For this review, take the finished solid that the model builds, in its own axes (mm). A direction names the side the tool comes from. Coordinates: 2 decimals unless noted, no trailing zeros. Loops run counter-clockwise (first coordinate to the right, second up) from the corner with the lowest first, then second, coordinate; pieces in that order, holes last.
```python
from build123d import *

# Parameters (mm, degrees)
EXTRUDE_1_DEPTH          = 2
SKETCH_2_R               = 1.5
CUT_EXTRUDE_1_DEPTH      = 56.208694967
MIRROR_2_COPY_1_SKETCH_R = 1.5
MIRROR_2_COPY_1_DEPTH    = 56.208694967
CUT_EXTRUDE_2_DEPTH      = 56.208694967
PATTERN_LINEAR_1_COUNT   = 6
PATTERN_LINEAR_1_PITCH   = 12
SKETCH_4_W               = 60
SKETCH_4_H               = 2
EXTRUDE_2_DEPTH          = 8
CUT_EXTRUDE_3_DEPTH      = 56.208694967
FILLET_1_R               = 3


with BuildPart() as part:
    # 草图1 → 凸台-拉伸1 (new body)
    with BuildSketch(Plane(origin=(0, 0, 0), x_dir=(1, 0, 0), z_dir=(0, 1, 0))):
        Polygon((-38, -30), (-38, -40), (38, -40), (38, -30), (30, -30), (30, 30), (38, 30), (38, 40), (-38, 40), (-38, 30), (-30, 30), (-30, -30), align=None)
    extrude(amount=EXTRUDE_1_DEPTH)

    # 草图2 → 切除-拉伸1 (cut, through all)
    with BuildSketch(Plane(origin=(0, 2, 0), x_dir=(1, 0, 0), z_dir=(0, 1, 0))):
        with Locations(Location((-34, 35, 0), (0, 0, 270))):
            Circle(SKETCH_2_R)
    cut_extrude_1 = extrude(amount=-CUT_EXTRUDE_1_DEPTH, mode=Mode.SUBTRACT)

    # 镜向1: 切除-拉伸1 across plane
    add(cut_extrude_1.mirror(Plane(origin=(0, 0, 0), x_dir=(0, 0, 1), z_dir=(1, 0, 0))), mode=Mode.SUBTRACT)

    # 镜向2: 切除-拉伸1 across plane
    add(cut_extrude_1.mirror(Plane.XY), mode=Mode.SUBTRACT)

    # 镜向2 copy 1 sketch → 镜向2 copy 1 (cut, through all)
    with BuildSketch(Plane(origin=(0, 2, 0), x_dir=(-1, 0, 0), z_dir=(0, 1, 0))):
        with Locations(Location((-34, 35, 0), (0, 0, 270))):
            Circle(MIRROR_2_COPY_1_SKETCH_R)
    extrude(amount=-MIRROR_2_COPY_1_DEPTH, mode=Mode.SUBTRACT)

    # 草图3 → 切除-拉伸2 (cut, through all)
    with BuildSketch(Plane(origin=(0, 2, 0), x_dir=(1, 0, 0), z_dir=(0, 1, 0))):
        with BuildLine():
            Line((-24, 34), (24, 34))
            ThreePointArc((24, 34), (28.5, 29.5), (24, 25))
            Line((24, 25), (-24, 25))
            ThreePointArc((-24, 25), (-28.5, 29.5), (-24, 34))
        make_face()
    cut_extrude_2 = extrude(amount=-CUT_EXTRUDE_2_DEPTH, mode=Mode.SUBTRACT)

    # 阵列(线性)1: 切除-拉伸2 ×6
    with Locations(*[(0, 0, i * PATTERN_LINEAR_1_PITCH) for i in range(1, PATTERN_LINEAR_1_COUNT)]):
        add(cut_extrude_2, mode=Mode.SUBTRACT)

    # 草图4 → 凸台-拉伸2 (add)
    with BuildSketch(Plane(origin=(30, 0, 0), x_dir=(0, 0, -1), z_dir=(1, 0, 0))):
        with Locations((0, 1)):
            Rectangle(SKETCH_4_W, SKETCH_4_H)
    extrude_2 = extrude(amount=EXTRUDE_2_DEPTH)

    # 镜向3: 凸台-拉伸2 across plane
    add(extrude_2.mirror(Plane(origin=(0, 0, 0), x_dir=(0, 0, 1), z_dir=(1, 0, 0))))

    # 草图6 → 切除-拉伸3 (cut, through all)
    with BuildSketch(Plane(origin=(0, 2, 0), x_dir=(1, 0, 0), z_dir=(0, 1, 0))):
        with BuildLine():
            Line((-38, 4), (-34, 4))
            ThreePointArc((-34, 4), (-30, 0), (-34, -4))
            Line((-34, -4), (-38, -4))
            Line((-38, -4), (-38, 4))
        make_face()
        with BuildLine():
            Line((38, -4), (38, 4))
            Line((38, 4), (34, 4))
            ThreePointArc((34, 4), (30, 0), (34, -4))
            Line((34, -4), (38, -4))
        make_face()
    extrude(amount=-CUT_EXTRUDE_3_DEPTH, mode=Mode.SUBTRACT)

    # 圆角1
    fillet_1_edges = [part.edges().sort_by_distance(p)[0] for p in [
        (-38, 1, 4),
        (-38, 1, -4),
        (38, 1, -4),
        (38, 1, 4),
        (38, 1, 40),
        (-38, 1, 40),
        (-38, 1, -40),
        (38, 1, -40),
    ]]
    fillet(fillet_1_edges, radius=FILLET_1_R)


solid = part.part
```
Q1. The part is to be moulded in two halves that separate along X. For faces 1 (the face through (30, 1, 0)), 2 (the face through (-37.1, 0.99, 4.86)), 3 (the face through (0, 1, -25)), say which applies: +X half, -X half, draft (parallel to the pull), parting line (faces both ways), or undercut.
Q2. Wall thickness on probe 1 along Z at (x, y) = (34, 1.45); probe 2 along X at (y, z) = (0.8, -35); probe 3 along X at (y, z) = (1.7, -26): over which ranges is each line inside the solid? List them lowest first.
Q3. Consider section C-C (y = 0.4). Count the separate pieces of the cut face and the enclosed holes in it, then the cut area to 3 significant figures.
Q4. Consider section B-B (x = -17.5). State the section outline as (y, z) points, then the cut area to 3 significant figures.
Q5. Consider section A-A (z = -29.5). State the section outline as (x, y) points.
Q6. For pin 1 Ø2.5 at (x, z) = (34, 35) entering from +Y, flat-tipped, find the tip position at first contact; note if it passes through.
Q7. Consider section D-D (z = 8.5). State the section outline as (x, y) points.
Q8. Machinability: for faces 4 (the face through (0, 1, 14)), 5 (the face through (37.1, 0.99, -4.86)), 6 (the face through (37.1, 1.01, -39.14)), which of the approach directions +Z, -Z, +X, -X, +Y, -Y give a long, thin tool a straight path to every point of the face, cutting with its end or side? Answer none if there is none.
Model answer:
1. face 1: +X half
1. face 2: -X half
1. face 3: undercut
2. probe 1: z = -40 to -36.5, -33.5 to -4, 4 to 33.5, 36.5 to 40
2. probe 2: x = -38 to -35.5, -32.5 to 32.5, 35.5 to 38
2. probe 3: x = -38 to -26.83, 26.83 to 38
3. separate pieces: 1
3. enclosed holes: 10
3. area: 2,950 mm2
4. outline: (0, -40) - (2, -40) - (2, -34) - (0, -34) - close; (0, -25) - (2, -25) - (2, -22) - (0, -22) - close; (0, -13) - (2, -13) - (2, -10) - (0, -10) - close; (0, -1) - (2, -1) - (2, 2) - (0, 2) - close; (0, 11) - (2, 11) - (2, 14) - (0, 14) - close; (0, 23) - (2, 23) - (2, 26) - (0, 26) - close; (0, 35) - (2, 35) - (2, 40) - (0, 40) - close
4. area: 52.0 mm2
5. outline: (-38, 0) - (-28.5, 0) - (-28.5, 2) - (-38, 2) - close; (28.5, 0) - (38, 0) - (38, 2) - (28.5, 2) - close
6. pin 1: passes through
7. outline: (-38, 0) - (-28.03, 0) - (-28.03, 2) - (-38, 2) - close; (28.03, 0) - (38, 0) - (38, 2) - (28.03, 2) - close
8. face 4: +Y, -Y
8. face 5: +X, +Y, -Y
8. face 6: -Z, +X, +Y, -Y
